from build123d import *

# Parameters (mm, degrees)
SKETCH_1_W          = 66
SKETCH_1_H          = 4.5
EXTRUDE_1_DEPTH     = 6
SKETCH_2_W          = 5.75
SKETCH_2_H          = 11
SKETCH_2_W_2        = 7
EXTRUDE_2_DEPTH     = 6
SKETCH_3_R          = 1.25
CUT_EXTRUDE_1_DEPTH = 51
SKETCH_4_R          = 1.5
CUT_EXTRUDE_2_DEPTH = 51
FILLET_1_R          = 2
FILLET_2_R          = 2
FILLET_3_R          = 2
FILLET_4_R          = 2
FILLET_5_R          = 2
FILLET_6_R          = 2
FILLET_7_R          = 2
FILLET_8_R          = 2
CHAMFER_1_SIZE      = 0.5
CHAMFER_2_SIZE      = 0.5


with BuildPart() as part:
    # 草图1 → 凸台-拉伸1 (new body)
    with BuildSketch(Plane(origin=(0, 0, 0), x_dir=(0, 0, -1), z_dir=(1, 0, 0))):
        Rectangle(SKETCH_1_W, SKETCH_1_H)
    extrude(amount=EXTRUDE_1_DEPTH)

    # 草图2 → 凸台-拉伸2 (add)
    with BuildSketch(Plane.ZY):
        with Locations((6.125, 7.75)):
            Rectangle(SKETCH_2_W, SKETCH_2_H)
        with Locations((19.5, 7.75)):
            Rectangle(SKETCH_2_W_2, SKETCH_2_H)
        with Locations((-19.5, 7.75)):
            Rectangle(SKETCH_2_W_2, SKETCH_2_H)
        with Locations((-6.125, 7.75)):
            Rectangle(SKETCH_2_W, SKETCH_2_H)
    extrude(amount=-EXTRUDE_2_DEPTH)

    # 草图3 → 切除-拉伸1 (cut)
    with BuildSketch(Plane.XY.offset(23)):
        with Locations((3, 8.182)):
            Circle(SKETCH_3_R)
    extrude(amount=-CUT_EXTRUDE_1_DEPTH, mode=Mode.SUBTRACT)

    # 草图4 → 切除-拉伸2 (cut)
    with BuildSketch(Plane(origin=(0, 2.25, 0), x_dir=(1, 0, 0), z_dir=(0, 1, 0))):
        with Locations((3, 0)):
            Circle(SKETCH_4_R)
        with Locations((3, 28)):
            Circle(SKETCH_4_R)
        with Locations((3, -28)):
            Circle(SKETCH_4_R)
    extrude(amount=-CUT_EXTRUDE_2_DEPTH, mode=Mode.SUBTRACT)

    # 圆角1
    fillet_1_edges = [part.edges().sort_by_distance(p)[0] for p in [
        (6, 13.25, 19.5),
    ]]
    fillet(fillet_1_edges, radius=FILLET_1_R)

    # 圆角2
    fillet_2_edges = [part.edges().sort_by_distance(p)[0] for p in [
        (6, 13.25, -19.5),
    ]]
    fillet(fillet_2_edges, radius=FILLET_2_R)

    # 圆角3
    fillet_3_edges = [part.edges().sort_by_distance(p)[0] for p in [
        (6, 13.25, 6.125),
    ]]
    fillet(fillet_3_edges, radius=FILLET_3_R)

    # 圆角4
    fillet_4_edges = [part.edges().sort_by_distance(p)[0] for p in [
        (6, 13.25, -6.125),
    ]]
    fillet(fillet_4_edges, radius=FILLET_4_R)

    # 圆角5
    fillet_5_edges = [part.edges().sort_by_distance(p)[0] for p in [
        (0, 13.25, -19.5),
    ]]
    fillet(fillet_5_edges, radius=FILLET_5_R)

    # 圆角6
    fillet_6_edges = [part.edges().sort_by_distance(p)[0] for p in [
        (0, 13.25, -6.125),
    ]]
    fillet(fillet_6_edges, radius=FILLET_6_R)

    # 圆角7
    fillet_7_edges = [part.edges().sort_by_distance(p)[0] for p in [
        (0, 13.25, 6.125),
    ]]
    fillet(fillet_7_edges, radius=FILLET_7_R)

    # 圆角8
    fillet_8_edges = [part.edges().sort_by_distance(p)[0] for p in [
        (0, 13.25, 19.5),
    ]]
    fillet(fillet_8_edges, radius=FILLET_8_R)

    # 倒角1
    chamfer_1_edges = [part.edges().sort_by_distance(p)[0] for p in [
        (3, 13.25, -16),
        (5.414213562, 12.664213562, -16),
        (0.585786438, 12.664213562, -16),
        (6, 6.75, -16),
        (0, 6.75, -16),
    ]]
    chamfer(chamfer_1_edges, length=CHAMFER_1_SIZE)

    # 倒角2
    chamfer_2_edges = [part.edges().sort_by_distance(p)[0] for p in [
        (0, 6.75, -23),
        (6, 6.75, -23),
        (0.585786438, 12.664213562, -23),
        (5.414213562, 12.664213562, -23),
        (3, 13.25, -23),
        (0, 6.75, -9),
        (6, 6.75, -9),
        (0.585786438, 12.664213562, -9),
        (5.414213562, 12.664213562, -9),
        (3, 13.25, -9),
        (0, 6.75, 3.25),
        (6, 6.75, 3.25),
        (0.585786438, 12.664213562, 3.25),
        (5.414213562, 12.664213562, 3.25),
        (3, 13.25, 3.25),
        (0, 6.75, 16),
        (6, 6.75, 16),
        (0.585786438, 12.664213562, 16),
        (5.414213562, 12.664213562, 16),
        (3, 13.25, 16),
        (0, 6.75, 23),
        (6, 6.75, 23),
        (0.585786438, 12.664213562, 23),
        (5.414213562, 12.664213562, 23),
        (3, 13.25, 23),
        (0, 6.75, 9),
        (6, 6.75, 9),
        (0.585786438, 12.664213562, 9),
        (5.414213562, 12.664213562, 9),
        (3, 13.25, 9),
        (0, 6.75, -3.25),
        (6, 6.75, -3.25),
        (0.585786438, 12.664213562, -3.25),
        (5.414213562, 12.664213562, -3.25),
        (3, 13.25, -3.25),
    ]]
    chamfer(chamfer_2_edges, length=CHAMFER_2_SIZE)


solid = part.part
Geometry check sheet. Reference: the model listing, model coordinates, mm. A direction names the side the tool comes from. Round coordinates to 2 decimals unless told otherwise and drop trailing zeros. Order: outer loops, then holes, each group sorted by start corner. A loop starts at its lowest first (then second) coordinate and runs counter-clockwise, first axis right, second up. Notation, with made-up numbers: M 71,8.5 L 85,8.5 A23 ccw 85,46.5 Z; hole C -30.5,63 d8. An arc over 180 degrees is marked long. Write each question's results on one line, items separated by ' | '. Start each with the question number.
1. Go/stop test with flat-tipped pins: P1, Ø2.5, axis at x = 3, z = 28, coming from the +Y side; P2, Ø2.5, axis at x = 3.5, y = 5, coming from the +Z side; P3, Ø2.5, axis at x = 3, y = 7.5, coming from the -Z side; P4, Ø3, axis at x = 2, z = -28.5, coming from the +Y side. Record where each tip stops, or that it passes through.
2. Material ranges on L1, parallel to Z at x = 3, y = 0.2; L2, parallel to Z at x = 5, y = 8.75; L3, parallel to Y at x = 3, z = 6.9, recorded low to high. Write a range as from..to.
3. Cross-section at B-B on z = 28. Record the boundary of the cut face in (x, y).
4. Draft check along Z on faces 1 (the face through (3, 6, 3.25)), 2 (the face through (3, 6, 23)), 3 (the face through (2.84, 9.42, 6.17)). Enter one of: pulls with the +Z half, pulls with the -Z half, needs draft (parallel to the pull), parting line crosses it, or undercut.
5. Cross-section at D-D on z = -5. Record the boundary of the cut face in (x, y), plus the area to 3 significant figures.
6. Cross-section at A-A on y = 10.5. Give the number of separate pieces and of enclosed holes in the cut face, plus the area to 3 significant figures.
7. Set-up check for faces 4 (the face through (3, 6, 9)), 5 (the face through (0.83, 12.4, -16.14)), 6 (the face through (5.144, 12.419, 16.135)): record each of +Z, -Z, +X, -X, +Y, -Y from which the full face is reachable in a straight line by a thin tool's end or side.
Resolved:
1) P1: through | P2: z = 23 | P3: z = -23 | P4: y = 2.25
2) L1: -33..-29.5, -26.5..-1.5, 1.5..26.5, 29.5..33 | L2: -23..-16, -9..-3.25, 3.25..9, 16..23 | L3: -2.25..6.93, 9.43..13.25
3) outline: M 0,-2.25 L 1.5,-2.25 L 1.5,2.25 L 0,2.25 Z; M 4.5,-2.25 L 6,-2.25 L 6,2.25 L 4.5,2.25 Z
4) face 1: undercut | face 2: pulls with the +Z half | face 3: needs draft
5) outline: M 0,-2.25 L 6,-2.25 L 6,11.25 A2 ccw 4,13.25 L 2,13.25 A2 ccw 0,11.25 Z; hole C 3,8.18 d2.5 | area: 86.4 mm2
6) separate pieces: 4 | enclosed holes: 0 | area: 151 mm2
7) face 4: +X, -X, +Y | face 5: -X, +Y | face 6: +X, +Y
